CAD build for the part. Positions are in the model's coordinates, mm. Face numbers are marked on the shaded views. A direction names the side the tool comes from. Coordinates: 2 decimals unless noted, no trailing zeros. Loops run counter-clockwise (first coordinate to the right, second up) from the corner with the lowest first, then second, coordinate; pieces in that order, holes last. Notation, with made-up numbers: (52, 2.5) -> (85, 2.5) arc R27 ccw to (85, 25.5) -> close; hole circle Ø2 at (-22, 7). An arc over 180 degrees is marked (long way). Write item = value, one per line. Start each with the question number.
(1) Pull direction Y, two halves, no side cores. Call the marked faces 1, 2, 3 and 4: +Y half, -Y half, draft (parallel to the pull), parting line (faces both ways), or undercut.
(2) Drill centre lines: line 1 (X direction, y = 12, z = -19); line 2 (Z direction, x = -31.75, y = 13.25) (3 decimals); line 3 (Z direction, x = 0, y = 14) (3 decimals). Where is each one in solid material? Low to high. Write a range as from..to.
(3) Flat gauge pins, fed straight in: P1, Ø3, axis at x = 12.5, y = 50, coming from the +Z side; P2, Ø1, axis at y = 26, z = 6, coming from the -X side; P3, Ø10, axis at y = 29.5, z = 2.5, coming from the +X side. Where does each tip first touch, or does it go through?
(4) Tool access for the marked faces 5, 6, 7, 8 and 9: list every direction of +Z, -Z, +X, -X, +Y, -Y with a clear straight run to the whole face (end or side of a thin tool).
(5) Band-saw the part on A-A (x = 30.5). Write the cut outline in (y, z).
(6) Band-saw the part on B-B (x = 0). Count the separate pieces of the cut face and the enclosed holes in it, and give its area (3 significant figures).
Autodesk Inventor part; units mm, degrees
sketch "Sketch1" plane through (0, 0, 0) normal (0, 1, 0) x (-1, 0, 0)
  line L0 (31.75, -25.4) -> (-31.75, -25.4)
  line L1 (-38.1, -19.05) -> (-38.1, 19.05)
  line L2 (-31.75, 25.4) -> (31.75, 25.4)
  line L3 (38.1, 19.05) -> (38.1, -19.05)
  arc A0 (38.1, 19.05) -> (31.75, 25.4) centre (31.75, 19.05) ccw
  arc A1 (31.75, -25.4) -> (38.1, -19.05) centre (31.75, -19.05) ccw
  arc A2 (-38.1, -19.05) -> (-31.75, -25.4) centre (-31.75, -19.05) ccw
  arc A3 (-31.75, 25.4) -> (-38.1, 19.05) centre (-31.75, 19.05) ccw
  circle A4 centre (31.75, -19.05) radius 3.175
  circle A5 centre (-31.75, -19.05) radius 3.175
  circle A6 centre (-31.75, 19.05) radius 3.175
  circle A7 centre (31.75, 19.05) radius 3.175
  line L4 (0, 25.4) -> (0, -25.4) construction
  line L5 (38.1, 0) -> (-38.1, 0) construction
  point P0 (0, 0)
  point P1 (0, 0)
  dimension "d0" = 6.35
  dimension "d1" = 6.35
  dimension "d2" = 76.2
  dimension "d3" = 50.8
  dimension "d4" = 38.1
  dimension "d5" = 25.4
extrude "MAIN BODY" add sketch "Sketch1" along normal blind 19.05
ref_plane "WP1" through (0, 0, 0) normal (0.5, 0, 0.866) x (0, 1, 0)
sketch "Sketch2" plane through (0, 0, 0) normal (0.5, 0, 0.866) x (0, 1, 0)
  line L0 (19.05, -40.1963) -> (19.05, 14.7963) construction
  line L1 (19.05, 19.05) -> (25.4, 19.05)
  line L2 (25.4, 19.05) -> (25.4, 12.7)
  line L3 (25.4, 12.7) -> (31.75, 12.7)
  line L4 (31.75, 12.7) -> (31.75, 19.05)
  line L5 (31.75, 19.05) -> (38.1, 19.05)
  line L6 (38.1, 19.05) -> (38.1, -19.05)
  line L7 (38.1, -19.05) -> (31.75, -19.05)
  line L8 (31.75, -19.05) -> (31.75, -12.7)
  line L9 (31.75, -12.7) -> (25.4, -12.7)
  line L10 (25.4, -12.7) -> (25.4, -19.05)
  line L11 (25.4, -19.05) -> (19.05, -19.05)
  line L12 (19.05, -19.05) -> (19.05, 19.05)
  arc A0 (38.1, -19.05) -> (38.1, 19.05) centre (38.1, 0) ccw
  circle A1 centre (38.1, 0) radius 9.525
  point P0 (0, 0)
  dimension "d9" = 19.05
  dimension "d10" = 6.35
  dimension "d11" = 6.35
  dimension "d13" = 6.35
  dimension "d14" = 6.35
  dimension "d15" = 38.1
  dimension "d17" = 19.05
  dimension "d18" = 6.35
  dimension "d19" = 6.35
  dimension "d20" = 19.05
extrude "TOP BOSS" add sketch "Sketch2" along normal mid plane 25.4 contours L1 L2 L3 L4 L5 L6 A1 L7 L8 L9 L10 L11 L12 | A0 L6 A1
sketch "Sketch6" plane through (0, 0, 0) normal (0, -1, 0) x (1, 0, 0)
  point P0 (0, 0)
  point P1 (0, 0)
hole "THROUGH HOLE" at (0, 0, 0) direction (0, 1, 0) diameter 6.35 end through all
equation "\"d11\" = d10"
equation "\"d13\" = d10"
equation "\"d14\" = d11"
equation "\"d18\" = d10"
equation "\"d19\" = d18"
properties part number "ANS9-TUT-BK" material "LCP Plastic"
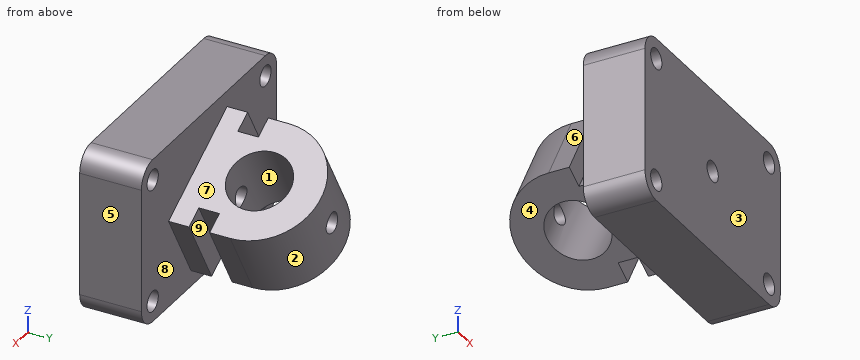
Findings below:
q1.face_1 = undercut
q1.face_2 = +Y half
q1.face_3 = -Y half
q1.face_4 = draft
q2.line_1 = -38.1..-34.92, -28.58..28.58, 34.92..38.1
q2.line_2 = -25.4..-22.225, -15.875..15.875, 22.225..25.4
q2.line_3 = -25.4..-3.175, 3.175..25.4
q3.P1 = 8.31
q3.P2 = -11.49
q3.P3 = 22.85
q4.face_5 = +Z, -Z, +X, +Y, -Y
q4.face_6 = +Z, -X, +Y
q4.face_7 = +Z, +X, +Y
q4.face_8 = +Y
q4.face_9 = -Z, +X
q5.outline = (0, -25.4) -> (19.05, -25.4) -> (19.05, -21.97) -> (0, -21.97) -> close; (0, -16.13) -> (19.05, -16.13) -> (19.05, 16.13) -> (0, 16.13) -> close; (0, 21.97) -> (19.05, 21.97) -> (19.05, 25.4) -> (0, 25.4) -> close
q6.separate_pieces = 4
q6.enclosed_holes = 0
q6.area = 1,330 mm²
